```python
from build123d import *

# Parameters (mm, degrees)
F0_W           = 190.5
F0_H           = 16.51
F1_DEPTH       = 4.7625
F2_R           = 4.7625
F3_DEPTH       = 57.15
F5_D           = 3.81
F5_CSINK_D     = 7.62
F5_CSINK_ANGLE = 90
F6_W           = 4.7625
F6_H           = 16.51
F7_DEPTH       = 3.175
F8_R           = 1.3462
F9_DEPTH       = 16.511


with BuildPart() as f1:
    # F0 (on Front) → F1 (new body)
    with BuildSketch(Plane.XZ):
        Rectangle(F0_W, F0_H)
    extrude(amount=F1_DEPTH)

    # F2 (on face) → F3 (join)
    with BuildSketch(Plane.XZ.offset(4.7625)):
        with Locations((-34.925, 1.27)):
            Circle(F2_R)
        with Locations((34.925, 1.27)):
            Circle(F2_R)
    extrude(amount=F3_DEPTH)

    # F5 (through all)
    with Locations(Plane.XZ.offset(4.7625)):
        with Locations((-76.2, 0), (76.2, 0)):
            CounterSinkHole(F5_D / 2, F5_CSINK_D / 2, counter_sink_angle=F5_CSINK_ANGLE)

    # F6 (on face) → F7 (cut)
    with BuildSketch(Plane.XZ.offset(4.7625)):
        Rectangle(F6_W, F6_H)
    extrude(amount=-F7_DEPTH, mode=Mode.SUBTRACT)

    # F8 (on face) → F9 (cut, through all)
    with BuildSketch(Plane.XY.offset(8.255)):
        with Locations((-34.925, -49.2125)):
            Circle(F8_R)
        with Locations((34.925, -49.2125)):
            Circle(F8_R)
    extrude(amount=-F9_DEPTH, mode=Mode.SUBTRACT)


solid = f1.part
```
Geometry check sheet. Reference: the model listing, model coordinates, mm. A direction names the side the tool comes from. Round coordinates to 2 decimals unless told otherwise and drop trailing zeros. Order: outer loops, then holes, each group sorted by start corner. A loop starts at its lowest first (then second) coordinate and runs counter-clockwise, first axis right, second up. Notation, with made-up numbers: M 28,49 L 45,49 A28 ccw 45,85 Z; hole C -27.5,20.25 d6. An arc over 180 degrees is marked long. Write item = value, one per line.
Q1. Set-up check for faces 1 (the cylindrical face through (39.468, -32.937, 2.701)), 2 (the flat face through (0, -1.588, 0)), 3 (the flat face through (-1, -1, -8.255)): record each of +Z, -Z, +X, -X, +Y, -Y from which the full face is reachable in a straight line by a thin tool's end or side.
Answer block:
face_1 = -Y
face_2 = +Z, -Z, -Y
face_3 = -Z, +X, -X, +Y, -Y
Q2. Section check A-A (x = -76.2). Enter the section's corners in (y, z) (1 decimal), plus the area to 3 significant figures.
Answer block:
outline = M -4.8,-8.3 L 0,-8.3 L 0,-1.9 L -2.9,-1.9 L -4.8,-3.8 Z; M -4.8,3.8 L -2.9,1.9 L 0,1.9 L 0,8.3 L -4.8,8.3 Z
area = 56.9 mm^2
Q3. Section check B-B (y = -28.5). Enter the section's corners in (x, z) (1 decimal), plus the area to 3 significant figures.
Answer block:
outline = C -34.9,1.3 d9.5; C 34.9,1.3 d9.5
area = 143 mm^2
Q4. Scan lines: line 1 (X direction, y = -1.15, z = 0) (3 decimals); line 2 (X direction, y = -1.7, z = 0) (3 decimals); line 3 (X direction, y = -25, z = 0.75). Record each from-to range of solid material in increasing order.
Answer block:
line_1 = -95.25 to -78.105, -74.295 to 74.295, 78.105 to 95.25
line_2 = -95.25 to -78.105, -74.295 to -2.381, 2.381 to 74.295, 78.105 to 95.25
line_3 = -39.66 to -30.19, 30.19 to 39.66
Q5. Depth check by flat-ended pin: pin 1 Ø6 at (y, z) = (-46, 2.5) entering from -X; pin 2 Ø1.5 at (y, z) = (-15, 5) entering from -X; pin 3 Ø1.4 at (x, z) = (-0.5, -3.5) entering from -Y; pin 4 Ø2 at (x, y) = (-34.92, -49.21) entering from +Z. Enter the tip coordinate at first touch or a pass-through.
Answer block:
pin_1 = -39.69
pin_2 = -38.64
pin_3 = -1.59
pin_4 = through
Q6. Release check for a two-part mould opening along Z. For faces 4 (the cylindrical face through (-39.683, -32.937, 1.479)), 5 (the cylindrical face through (-74.297, -1.409, 0.084)), 6 (the flat face through (35, -61.912, 1)) record: released by +Z, released by -Z, zero draft, split by the parting line, or undercut.
Answer block:
face_4 = split by the parting line
face_5 = undercut
face_6 = zero draft
Q7. Section check C-C (x = 62). Enter the section's corners in (y, z) (1 decimal).
Answer block:
outline = M -4.8,-8.3 L 0,-8.3 L 0,8.3 L -4.8,8.3 Z
